Input: part model. Units: mm. Frame: model coordinates. A direction names the side the tool comes from. Give positions to 0.01 mm unless a question says otherwise; leave off trailing zeros. Write each loop counter-clockwise with the first axis right and the second up, starting at its lowest first coordinate (ties: lowest second). Pieces come first, ordered by that corner, then holes. Notation, with made-up numbers: (-35, 37.5) - (12, 37.5) arc R35 cw to (12, 71.5) - close; hole circle Ø3 at (79.5, 24.5). An arc over 180 degrees is marked (long way). Answer as a JSON object with one key per item and string values. Group by question number.
Autodesk Inventor part; units mm, degrees
ref_plane "YZ Plane" through (0, 0, 0) normal (1, 0, 0) x (0, 1, 0)
ref_plane "XZ Plane" through (0, 0, 0) normal (0, 1, 0) x (-1, 0, 0)
ref_plane "XY Plane" through (0, 0, 0) normal (0, 0, 1) x (1, 0, 0)
sketch "Sketch1" plane through (0, 0, 0) normal (0, 1, 0) x (-1, 0, 0)
  line L0 (0, 0) -> (71.12, 0)
  line L1 (71.12, 0) -> (71.12, 40.64)
  line L2 (71.12, 40.64) -> (0, 40.64)
  line L3 (0, 40.64) -> (0, 0)
  dimension "d0" = 71.12
  dimension "d1" = 40.64
extrude "Extrusion1" add sketch "Sketch1" along normal blind 2.54
sketch "Sketch8" plane through (0, 2.54, 0) normal (0, 1, 0) x (1, 0, 0)
  line L0 (0, -40.64) -> (0, 0)
  circle A0 centre (-6.35, -37.719) radius 0.8
  circle A1 centre (-6.35, -2.921) radius 0.8
  circle A2 centre (-57.15, -2.921) radius 0.8
  circle A3 centre (-57.15, -37.719) radius 0.8
  dimension "d75" = 1.6
  dimension "d76" = 1.6
  dimension "d77" = 1.6
  dimension "d78" = 1.6
  dimension "d79" = 6.35
  dimension "d108" = 50.8
hole "Hole2" at (-57.15, 2.54, 2.921) at (-57.15, 2.54, 37.719) at (-6.35, 2.54, 37.719) at (-6.35, 2.54, 2.921) direction (0, -1, 0) diameter 1.6 end through all counterbore diameter 3.5 counterbore depth 1.27
sketch "Sketch9" plane through (0, 2.54, 0) normal (0, 1, 0) x (1, 0, 0)
  line L0 (0, 0) -> (-71.12, 0)
  line L1 (-71.12, 0) -> (-71.12, -40.64)
  line L2 (0, -40.64) -> (0, 0)
  arc A0 (0, -39.0525) -> (-1.5875, -40.64) centre (0, -40.64) ccw
  arc A1 (-1.5875, 0) -> (0, -1.5875) centre (0, 0) ccw
  arc A2 (-69.5325, -40.64) -> (-71.12, -39.0525) centre (-71.12, -40.64) ccw
  arc A3 (-71.12, -1.5875) -> (-69.5325, 0) centre (-71.12, 0) ccw
  line L3 (-1.5875, 0) -> (0, 0)
  line L4 (0, 0) -> (0, -1.5875)
  line L5 (0, -39.0525) -> (0, -40.64)
  line L6 (0, -40.64) -> (-1.5875, -40.64)
  line L7 (-69.5325, -40.64) -> (-71.12, -40.64)
  line L8 (-71.12, -40.64) -> (-71.12, -39.0525)
  line L9 (-69.5325, 0) -> (-71.12, 0)
  line L10 (-71.12, 0) -> (-71.12, -1.5875)
  point P0 (-69.85, -7.9375)
  dimension "d87" = 1.5875
  dimension "d89" = 1.5875
  dimension "d90" = 1.5875
  dimension "d91" = 1.5875
extrude "Extrusion9" cut sketch "Sketch9" against normal through all
sketch "Sketch10" plane through (0, 2.54, 0) normal (0, 1, 0) x (1, 0, 0)
  circle A0 centre (-13.4874, -15.5956) radius 3.175
  circle A1 centre (-13.4874, -25.0444) radius 3.175
  line L0 (0, -39.0525) -> (0, -1.5875)
  line L1 (-1.5875, 0) -> (-69.5325, 0)
  dimension "d95" = 6.35
  dimension "d96" = 6.35
  dimension "d122" = 13.4874
  dimension "d123" = 13.4874
  dimension "d125" = 9.4488
  dimension "d126" = 15.5956
extrude "Extrusion10" add sketch "Sketch10" along normal blind 6.35
sketch "Sketch11" plane through (-13.4874, 8.89, 15.5956) normal (0, 1, 0) x (1, 0, 0)
  circle A0 centre (0, 0) radius 3.175
  circle A1 centre (0, -9.4488) radius 3.175
  circle A2 centre (0, 0) radius 0.875
  circle A3 centre (0, -9.4488) radius 0.875
  line L0 (0, -12.6238) -> (17.5736, -12.6238)
  point P0 (13.4874, 15.5956)
  dimension "d106" = 1.75
  dimension "d107" = 1.75
sketch "Sketch12" plane through (0, 2.54, 0) normal (0, 1, 0) x (1, 0, 0)
  line L0 (-71.12, -1.5875) -> (-71.12, -39.0525)
  line L1 (-71.12, 2.2213) -> (-59.1056, 2.2213)
  line L2 (-59.1056, -41.9087) -> (-71.12, -41.9087)
  line L3 (-71.12, -41.9087) -> (-71.12, 2.2213)
  line L4 (0, -39.0525) -> (0, -1.5875)
  line L5 (-59.1056, -41.9087) -> (-52.7556, -41.9087)
  line L6 (-52.7556, -41.9087) -> (-52.7556, -21.2712)
  line L7 (-52.7556, -21.2712) -> (-59.1056, -21.2712)
  line L8 (-59.1056, 2.2213) -> (-59.1056, -21.2712)
  dimension "d128" = 20.6375
  dimension "d129" = 6.35
extrude "Extrusion11" cut sketch "Sketch12" against normal blind 25.4
extrude "Extrusion12" cut sketch "Sketch11" against normal blind 5 contours A2 | A3
properties part number "CustomBox_ardplate"
1) Pin query (flat end, axial travel): P1, Ø1.5, axis at x = -46.5, z = 20.5, coming from the -Y side; P2, Ø4, axis at x = -6, z = 2, coming from the +Y side; P3, Ø1.3, axis at y = 1.5, z = 35.5, coming from the -X side; P4, Ø2, axis at x = -57.15, z = 2.921, coming from the +Y side. Return the tip coordinate at first contact, or that it passes through.
2) Reachability of faces 1 (the face through (-1.135, 1.288, 1.11)), 2 (the face through (-52.756, 1, 31)), 3 (the face through (-15.83, 5.67, 17.74)) from +Z, -Z, +X, -X, +Y, -Y: full face, straight path, thin tool, end or side. Return the list, or none.
3) Cut plane A-A on x = -6.35. Return the cut outline in (y, z).
4) Mould query, pull axis X, two halves, no side actions, for faces 4 (the face through (-5.57, 0.63, 2.75)), 5 (the face through (-12.8, 8.89, 14.8)), 6 (the face through (-14.176, 5.671, 21.945)), 7 (the face through (-6, 1.27, 4)). Classes: +X half, -X half, draft (parallel to the pull), parting line (faces both ways), or undercut.
5) Cut plane D-D on z = 31. Return the cut outline in (x, y), and give its area (3 significant figures).
6) Cut plane B-B on x = -57.15. Return the cut outline in (y, z), and give its area (3 significant figures).
7) Cut plane C-C on y = 5. Return the cut outline in (x, z) (3 decimals).
8) Line query: line 1 along Z through (x, y) = (-6.35, 0.85); line 2 along Z through (x, y) = (-6.35, 1.9); line 3 along Z through (x, y) = (-57.15, 0.8). Output: solid intervals per line, ascending. Write a range as from..to.
Filled in:
{
 "1": {"P1": "stops at y = 0", "P2": "stops at y = 2.54", "P3": "stops at x = -52.76", "P4": "stops at y = 1.27"},
 "2": {"face 1": "-Z, +X, +Y, -Y", "face 2": "+Z, -X, +Y, -Y", "face 3": "+Y"},
 "3": {"outline": "(0, 0) - (2.54, 0) - (2.54, 1.17) - (1.27, 1.17) - (1.27, 2.12) - (0, 2.12) - close; (0, 3.72) - (1.27, 3.72) - (1.27, 4.67) - (2.54, 4.67) - (2.54, 35.97) - (1.27, 35.97) - (1.27, 36.92) - (0, 36.92) - close; (0, 38.52) - (1.27, 38.52) - (1.27, 39.47) - (2.54, 39.47) - (2.54, 40.64) - (0, 40.64) - close"},
 "4": {"face 4": "undercut", "face 5": "draft", "face 6": "parting line", "face 7": "undercut"},
 "5": {"outline": "(-52.76, 0) - (0, 0) - (0, 2.54) - (-52.76, 2.54) - close", "area": "134 mm²"},
 "6": {"outline": "(0, 0) - (2.54, 0) - (2.54, 1.17) - (1.27, 1.17) - (1.27, 2.12) - (0, 2.12) - close; (0, 3.72) - (1.27, 3.72) - (1.27, 4.67) - (2.54, 4.67) - (2.54, 21.27) - (0, 21.27) - close", "area": "47.6 mm²"},
 "7": {"outline": "circle Ø6.35 at (-13.487, 15.596); circle Ø6.35 at (-13.487, 25.044); hole circle Ø1.75 at (-13.487, 15.596); hole circle Ø1.75 at (-13.487, 25.044)"},
 "8": {"line 1": "z = 0..2.12, 3.72..36.92, 38.52..40.64", "line 2": "z = 0..1.17, 4.67..35.97, 39.47..40.64", "line 3": "z = 0..2.12, 3.72..21.27"}
}
